```python
from build123d import *

# Parameters (mm, degrees)
SKETCH_1_R               = 72.1
SKETCH_1_R_2             = 65.1
EXTRUDE_1_DEPTH          = 13
SKETCH_2_R               = 2.1
CUT_EXTRUDE_1_DEPTH      = 13
PATTERN_CIRCULAR_1_COUNT = 10


with BuildPart() as part:
    # 草图1 → 凸台-拉伸1 (new body)
    with BuildSketch(Plane(origin=(0, 0, 0), x_dir=(1, 0, 0), z_dir=(0, 1, 0))):
        with Locations(Location((0, 0, 0), (0, 0, 90))):
            Circle(SKETCH_1_R)
        with Locations(Location((0, 0, 0), (0, 0, 90))):
            Circle(SKETCH_1_R_2, mode=Mode.SUBTRACT)
    extrude(amount=EXTRUDE_1_DEPTH)

    # 草图2 → 切除-拉伸1 (cut)
    with BuildSketch(Plane(origin=(0, 13, 0), x_dir=(1, 0, 0), z_dir=(0, 1, 0))):
        with Locations((-72.1, 0)):
            Circle(SKETCH_2_R)
    cut_extrude_1 = extrude(amount=-CUT_EXTRUDE_1_DEPTH, mode=Mode.SUBTRACT)

    # 阵列(圆周)1: 切除-拉伸1 ×10 about axis
    pattern_circular_1_axis = Axis((0, 0, 0), (0, 1, 0))
    for i in range(1, PATTERN_CIRCULAR_1_COUNT):
        add(cut_extrude_1.rotate(pattern_circular_1_axis, i * 360 / PATTERN_CIRCULAR_1_COUNT), mode=Mode.SUBTRACT)


solid = part.part
```
Geometry: final body of the model. Coordinates: model frame, mm. Coordinates: 2 decimals unless noted, no trailing zeros. Order: outer loops, then holes, each group sorted by start corner. A loop starts at its lowest first (then second) coordinate and runs counter-clockwise, first axis right, second up. Notation, with made-up numbers: (18.25, 30.25) -> (63.25, 30.25) arc R11 cw to (63.25, 48.25) -> close; hole circle Ø7 at (45, 54.25). An arc over 180 degrees is marked (long way). Write each question's results on one line, items separated by ' | '. Start each with the question number.
1) Material intervals for line 1 along Z through (x, y) = (-58.5, 9.75); line 2 along Z through (x, y) = (41, 2.5); line 3 along X through (y, z) = (3.5, -28), sorted ascending.
2) Cut plane C-C, the plane y = 2.5. Output: boundary loops of the cut face in (x, z), and give its area (3 significant figures).
3) Mould query, pull axis X, two halves, no side actions, for faces 1 (the cylindrical face through (0.3, 6.4, -72.1)), 2 (the cylindrical face through (70, 7, 0)), 3 (the cylindrical face through (21.67, 6.59, 66.56)). Classes: released by +X, released by -X, zero draft, split by the parting line, or undercut.
4) First-contact query: pin 1 (5 mm diameter, centred on y = 8.5, z = -26, fed in from -X); pin 2 (1 mm diameter, centred on y = 6, z = -53.5, fed in from -X); pin 3 (1 mm diameter, centred on x = 15.5, y = 10, fed in from -Z). Flat tips, straight axial feed; report the tip coordinate or a pass-through.
5) Cut plane A-A, the plane z = 0. Output: boundary loops of the cut face in (x, y), and give its area (3 significant figures).
6) Cut plane B-B, the plane x = 0. Output: boundary loops of the cut face in (y, z).
Checks:
1) line 1: -40.29 to -28.56, 28.56 to 40.29 | line 2: -59.31 to -50.57, 50.57 to 59.31 | line 3: -66.44 to -58.77, 58.77 to 66.44
2) outline: (-72.07, -2.1) arc R72.1 ccw to (-59.54, -40.66) arc R2.1 cw to (-57.07, -44.06) arc R72.1 ccw to (-24.27, -67.89) arc R2.1 cw to (-20.27, -69.19) arc R72.1 ccw to (20.27, -69.19) arc R2.1 cw to (24.27, -67.89) arc R72.1 ccw to (57.07, -44.06) arc R2.1 cw to (59.54, -40.66) arc R72.1 ccw to (72.07, -2.1) arc R2.1 cw to (72.07, 2.1) arc R72.1 ccw to (59.54, 40.66) arc R2.1 cw to (57.07, 44.06) arc R72.1 ccw to (24.27, 67.89) arc R2.1 cw to (20.27, 69.19) arc R72.1 ccw to (-20.27, 69.19) arc R2.1 cw to (-24.27, 67.89) arc R72.1 ccw to (-57.07, 44.06) arc R2.1 cw to (-59.54, 40.66) arc R72.1 ccw to (-72.07, 2.1) arc R2.1 cw to start; hole circle Ø130.2 at (0, 0) | area: 2,950 mm^2
3) face 1: split by the parting line | face 2: released by +X | face 3: undercut
4) pin 1: x = -68.16 | pin 2: x = -48.88 | pin 3: z = -70.52
5) outline: (-70, 0) -> (-65.1, 0) -> (-65.1, 13) -> (-70, 13) -> close; (65.1, 0) -> (70, 0) -> (70, 13) -> (65.1, 13) -> close | area: 127 mm^2
6) outline: (0, -72.1) -> (13, -72.1) -> (13, -65.1) -> (0, -65.1) -> close; (0, 65.1) -> (13, 65.1) -> (13, 72.1) -> (0, 72.1) -> close
